Source: CAD feature listing. Evaluate the final solid. Frame: model axes, mm. Face numbers are marked on the shaded views. A direction names the side the tool comes from. Give positions to 0.01 mm unless a question says otherwise; leave off trailing zeros. Order: outer loops, then holes, each group sorted by start corner. A loop starts at its lowest first (then second) coordinate and runs counter-clockwise, first axis right, second up. Notation, with made-up numbers: M 78,81.25 L 127,81.25 A14 cw 127,89.25 Z; hole C -28.5,83.5 d7. An arc over 180 degrees is marked long. Answer as a JSON object with one key per item and string values. Group by question number.
1. Section query A-A (z = -47). Output: boundary loops of the cut face in (x, y).
2. Pin query (flat end, axial travel): P1, Ø10, axis at x = 72, z = -18, coming from the -Y side. Return the tip coordinate at first contact, or that it passes through.
3. Pull-direction query (X, two-part tool) for the marked faces 3, 4, 5 and 6; classes: +X half, -X half, draft (parallel to the pull), parting line (faces both ways), or undercut.
4. Set-up query: the marked faces 1 and 2. Return all of +Z, -Z, +X, -X, +Y, -Y with unobstructed straight access to the full face (end or side cutting, diameter ignored); none if empty.
5. Section query B-B (x = 48). Output: boundary loops of the cut face in (y, z), plus the area to 3 significant figures.
6. Material intervals for L1, parallel to Z at x = 20, y = -53; L2, parallel to X at y = -60, z = 47; L3, parallel to Y at x = -36, z = 19, sorted ascending. Write a range as [from, to].
7. Section query C-C (y = -79.5). Output: boundary loops of the cut face in (x, z).
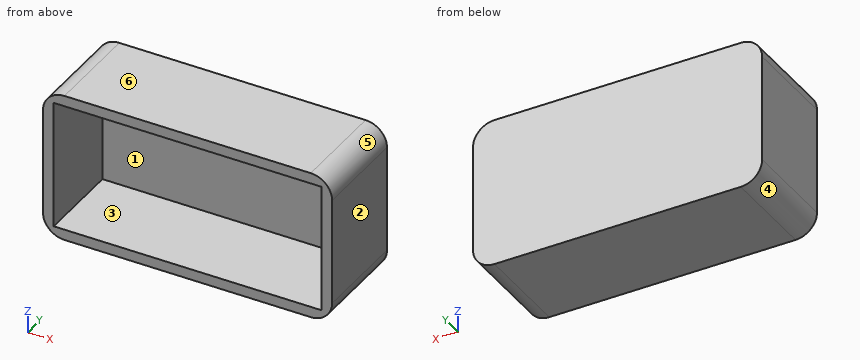
from build123d import *

# Parameters (mm, degrees)
F0_W     = 270
F0_H     = 140
F1_DEPTH = 90
F2_W     = 250
F2_H     = 120
F3_DEPTH = 80
F4_R     = 20


with BuildPart() as f1:
    # F0 (on Front) → F1 (new body)
    with BuildSketch(Plane.XZ):
        Rectangle(F0_W, F0_H)
    extrude(amount=F1_DEPTH)

    # F2 (on face) → F3 (cut)
    with BuildSketch(Plane.XZ.offset(90)):
        Rectangle(F2_W, F2_H)
    extrude(amount=-F3_DEPTH, mode=Mode.SUBTRACT)

    # F4
    f4_edges = [f1.edges().sort_by_distance(p)[0] for p in [
        (-135, -45, 70),
        (135, -45, 70),
        (-135, -45, -70),
        (135, -45, -70),
    ]]
    fillet(f4_edges, radius=F4_R)


solid = f1.part
Answer sheet:
{
 "1": {"outline": "M -135,-90 L -125,-90 L -125,-10 L 125,-10 L 125,-90 L 135,-90 L 135,0 L -135,0 Z"},
 "2": {"P1": "y = -10"},
 "3": {"face 3": "undercut", "face 4": "-X half", "face 5": "+X half", "face 6": "draft"},
 "4": {"face 1": "-Y", "face 2": "+Z, -Z, +X, +Y, -Y"},
 "5": {"outline": "M -90,-70 L 0,-70 L 0,70 L -90,70 L -90,60 L -10,60 L -10,-60 L -90,-60 Z", "area": "3,000 mm^2"},
 "6": {"L1": "[-70, -60], [60, 70]", "L2": "[-135, -125], [125, 135]", "L3": "[-10, 0]"},
 "7": {"outline": "M -135,-50 A20 ccw -115,-70 L 115,-70 A20 ccw 135,-50 L 135,50 A20 ccw 115,70 L -115,70 A20 ccw -135,50 Z; hole M -125,-60 L 125,-60 L 125,60 L -125,60 Z"}
}
